Geometry: see drawing. Coordinates: mm, zero at the bounding-box minimum. A direction names the side the tool comes from. Coordinates: 2 decimals unless noted, no trailing zeros. Write each loop counter-clockwise with the first axis right and the second up, starting at its lowest first coordinate (ties: lowest second). Pieces come first, ordered by that corner, then holes.
1) Section query A-A (z = 5.25). Output: boundary loops of the cut face in (x, y), then the cut area to 3 significant figures.
2) Draft query along Y for the marked faces 5, 6 and 7. Return one class per face: pulls with the +Y half, pulls with the -Y half, needs draft (parallel to the pull), parting line crosses it, or undercut.
3) Section query D-D (z = 10.5). Output: boundary loops of the cut face in (x, y), then the cut area to 3 significant figures.
4) Line query: L1, parallel to Y at x = 20.5, z = 6; L2, parallel to Z at x = 27, y = 19.75; L3, parallel to X at y = 18.5, z = 10.25. Output: solid intervals per line, ascending.
5) Section query C-C (x = 27). Output: boundary loops of the cut face in (y, z), then the cut area to 3 significant figures.
6) Section query B-B (y = 16). Output: boundary loops of the cut face in (x, z), then the cut area to 3 significant figures.
7) Set-up query: the marked faces 1, 2, 3 and 4. Return all of +Z, -Z, +X, -X, +Y, -Y with unobstructed straight access to the full face (end or side cutting, diameter ignored); none if empty.
8) Pin query (flat end, axial travel): pin 1 Ø3 at (y, z) = (10, 5.5) entering from +X; pin 2 Ø4.5 at (x, z) = (24.5, 10.5) entering from -Y; pin 3 Ø6.5 at (y, z) = (9.5, 6) entering from -X; pin 4 Ø7 at (y, z) = (6, 6) entering from +X. Return the tip coordinate at first contact, or that it passes through.
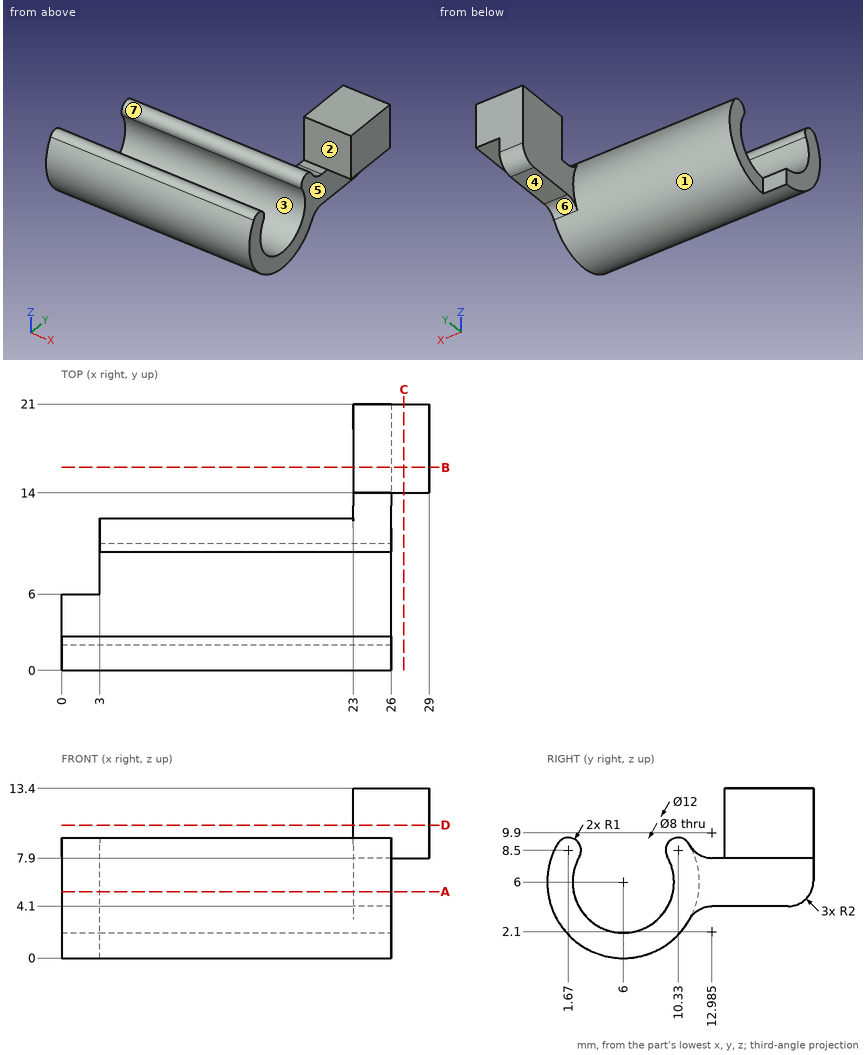
Answer:
1. outline: (0, 0.05) - (26, 0.05) - (26, 2.07) - (0, 2.07) - close; (3, 9.93) - (26, 9.93) - (26, 20.81) - (23, 20.81) - (23, 11.95) - (3, 11.95) - close
1. area: 126 mm2
2. face 5: needs draft
2. face 6: pulls with the +Y half
2. face 7: undercut
3. outline: (23, 14) - (29, 14) - (29, 21) - (23, 21) - close
3. area: 42.0 mm2
4. L1: y = 0 to 2, 10 to 12
4. L2: z = 7.9 to 13.4
4. L3: x = 23 to 29
5. outline: (14, 7.9) - (21, 7.9) - (21, 13.4) - (14, 13.4) - close
5. area: 38.5 mm2
6. outline: (23, 4.1) - (26, 4.1) - (26, 7.9) - (29, 7.9) - (29, 13.4) - (23, 13.4) - close
6. area: 44.4 mm2
7. face 1: -X
7. face 2: +Z, +X, -X
7. face 3: +X, -X
7. face 4: -Z, +X, -X, +Y
8. pin 1: stops at x = 26
8. pin 2: stops at y = 0.44
8. pin 3: stops at x = 3
8. pin 4: passes through
